from build123d import *

# Parameters (mm, degrees)
AUFSATZ_LINEAR_AUSTRAGEN1_DEPTH                      = 4
FORMSENKUNG_F_R_M3_SENKSCHRAUBE_MIT_INNE_D           = 2
FORMSENKUNG_F_R_M3_SENKSCHRAUBE_MIT_INNE_CSINK_D     = 3.5
FORMSENKUNG_F_R_M3_SENKSCHRAUBE_MIT_INNE_CSINK_ANGLE = 90


with BuildPart() as part:
    # Skizze1 → Aufsatz-Linear austragen1 (new body, symmetric)
    with BuildSketch(Plane.XY):
        Polygon((-31.9, 0), (-15.9, 0), (-15.9, 0.8), (15.9, 0.8), (15.9, 0), (31.9, 0), (31.9, -3), (-31.9, -3), align=None)
    extrude(amount=AUFSATZ_LINEAR_AUSTRAGEN1_DEPTH, both=True)

    # Formsenkung für M3 Senkschraube mit Innensechskant1 (through all)
    with Locations(Plane(origin=(0, -3, 0), x_dir=(-1, 0, 0), z_dir=(0, -1, 0))):
        with Locations((8, 0), (-8, 0)):
            CounterSinkHole(FORMSENKUNG_F_R_M3_SENKSCHRAUBE_MIT_INNE_D / 2, FORMSENKUNG_F_R_M3_SENKSCHRAUBE_MIT_INNE_CSINK_D / 2, counter_sink_angle=FORMSENKUNG_F_R_M3_SENKSCHRAUBE_MIT_INNE_CSINK_ANGLE)


solid = part.part
For this review, take the finished solid that the model builds, in its own axes (mm). A direction names the side the tool comes from. Give positions to 0.01 mm unless a question says otherwise; leave off trailing zeros. Order: outer loops, then holes, each group sorted by start corner. A loop starts at its lowest first (then second) coordinate and runs counter-clockwise, first axis right, second up. Notation, with made-up numbers: (32, -6.75) - (47, -6.75) arc R3 cw to (47, -1.75) - close; hole circle Ø9 at (-16, 69). An arc over 180 degrees is marked (long way). Answer as a JSON object with one key per item and string values. Group by question number.
Item 1: Clearance check with flat-ended pins moving along their axes: pin 1 Ø3 at (x, z) = (8, 0) entering from -Y; pin 2 Ø1.6 at (x, z) = (-8, 0) entering from +Y; pin 3 Ø0.6 at (y, z) = (0.5, 0.5) entering from -X. State where each tip first meets the part, or that it passes through.
Item 2: Take a section at B-B on z = 0. Give the boundary of the cut face in (x, y).
Item 3: Machinability: for faces 4 (the flat face through (24, 0, 0)), 5 (the flat face through (-24, 0, 0)), 6 (the cylindrical face through (7.2, -0.7, 0.6)), which of the approach directions +Z, -Z, +X, -X, +Y, -Y give a long, thin tool a straight path to every point of the face, cutting with its end or side? Answer none if there is none.
Item 4: Draft analysis for pull direction X (two halves, no side actions). For faces 1 (the flat face through (0, 0.8, 0)), 2 (the flat face through (-31.9, -2, 0)), 3 (the cylindrical face through (-8.8, -0.7, 0.6)), state which applies: pulls with the +X half, pulls with the -X half, needs draft (parallel to the pull), parting line crosses it, or undercut.
Item 5: Take a section at A-A on x = -8. Give the boundary of the cut face in (y, z).
Item 6: Wall thickness on line 1 along Z through (x, y) = (-8, -1.5); line 2 along X through (y, z) = (-1.35, 0.5); line 3 along Y through (x, z) = (26, -1.5): over which ranges is each line inside the solid? List them lowest first.
Item 7: Take a section at C-C on x = -25. Give the boundary of the cut face in (y, z), and give its area (3 significant figures).
Reported:
{
 "1": {"pin 1": "y = -2.75", "pin 2": "through", "pin 3": "x = -15.9"},
 "2": {"outline": "(-31.9, -3) - (-9.75, -3) - (-9, -2.25) - (-9, 0.8) - (-15.9, 0.8) - (-15.9, 0) - (-31.9, 0) - close; (-7, -2.25) - (-6.25, -3) - (6.25, -3) - (7, -2.25) - (7, 0.8) - (-7, 0.8) - close; (9, -2.25) - (9.75, -3) - (31.9, -3) - (31.9, 0) - (15.9, 0) - (15.9, 0.8) - (9, 0.8) - close"},
 "3": {"face 4": "+Z, -Z, +X, +Y", "face 5": "+Z, -Z, -X, +Y", "face 6": "+Y, -Y"},
 "4": {"face 1": "needs draft", "face 2": "pulls with the -X half", "face 3": "undercut"},
 "5": {"outline": "(-3, -4) - (0.8, -4) - (0.8, -1) - (-2.25, -1) - (-3, -1.75) - close; (-3, 1.75) - (-2.25, 1) - (0.8, 1) - (0.8, 4) - (-3, 4) - close"},
 "6": {"line 1": "-4 to -1, 1 to 4", "line 2": "-31.9 to -8.87, -7.13 to 7.13, 8.87 to 31.9", "line 3": "-3 to 0"},
 "7": {"outline": "(-3, -4) - (0, -4) - (0, 4) - (-3, 4) - close", "area": "24.0 mm^2"}
}
